Part print with two shaded views. Sizes in mm from the minimum x, y, z corner. A direction names the side the tool comes from. Round coordinates to 2 decimals unless told otherwise and drop trailing zeros. Loops run counter-clockwise (first coordinate to the right, second up) from the corner with the lowest first, then second, coordinate; pieces in that order, holes last. Notation, with made-up numbers: (61.5, 11.5) - (75.5, 11.5) arc R17 ccw to (75.5, 22.5) - close; hole circle Ø8 at (-37, 77). An arc over 180 degrees is marked (long way). Write each question's results on one line, items separated by ' | '. Start each with the question number.
(1) Flat gauge pins, fed straight in: P1, Ø3, axis at x = 16, z = 3.5, coming from the +Y side (1 decimal); P2, Ø1, axis at x = 13.5, y = 4.5, coming from the -Z side; P3, Ø3, axis at y = 3, z = 8, coming from the +X side. Where does each tip first touch, or does it go through?
(2) Drill centre lines: L1, parallel to X at y = 2.25, z = 2; L2, parallel to Y at x = 11, z = 6; L3, parallel to Y at x = 18, z = 7.25. Where is each one in solid material? Low to high.
(3) Cut at A-A, the plane z = 6. List the corners of the cut face in (x, y).
(4) Cut at C-C, the plane y = 1.5. List the corners of the cut face in (x, z).
(5) Cut at D-D, the plane z = 1. List the corners of the cut face in (x, y), then the cut area to 3 significant figures.
(6) Tool access for the marked faces 1 and 2: list every direction of +Z, -Z, +X, -X, +Y, -Y with a clear straight run to the whole face (end or side of a thin tool).
(7) Cut at B-B, the plane x = 36. List the corners of the cut face in (y, z).
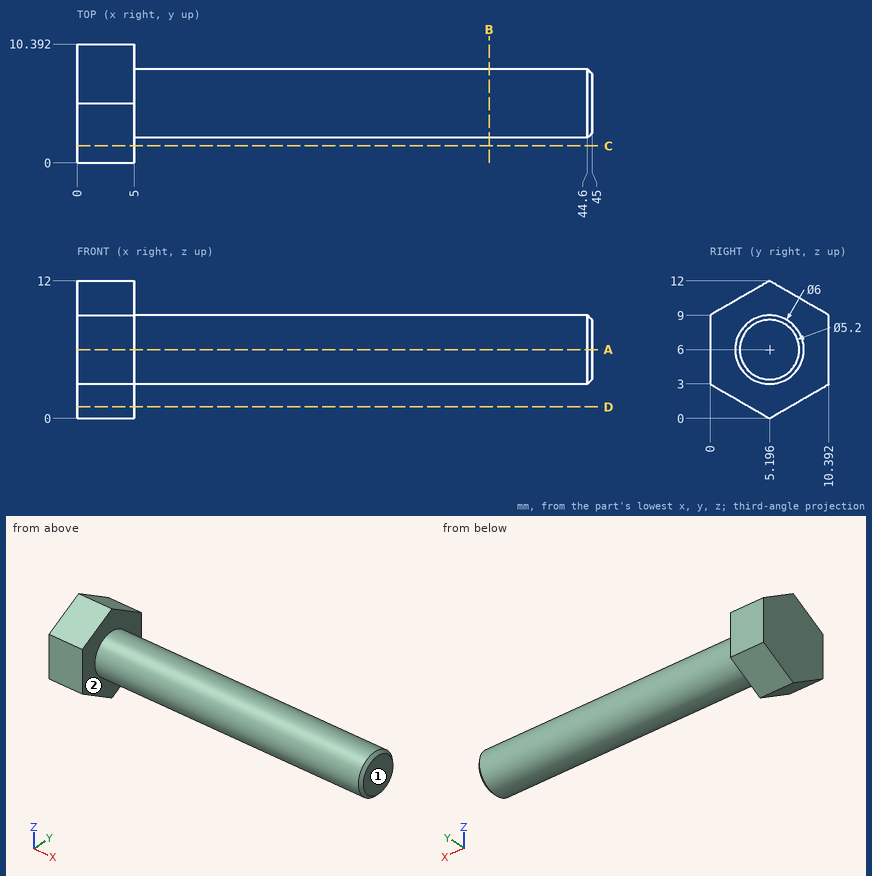
A:
1) P1: y = 8 | P2: z = 3.01 | P3: x = 45
2) L1: 0 to 5 | L2: 2.2 to 8.2 | L3: 2.47 to 7.92
3) outline: (0, 0) - (5, 0) - (5, 2.2) - (44.6, 2.2) - (45, 2.6) - (45, 7.8) - (44.6, 8.2) - (5, 8.2) - (5, 10.39) - (0, 10.39) - close
4) outline: (0, 2.13) - (5, 2.13) - (5, 9.87) - (0, 9.87) - close
5) outline: (0, 3.46) - (5, 3.46) - (5, 6.93) - (0, 6.93) - close | area: 17.3 mm2
6) face 1: +Z, -Z, +X, +Y, -Y | face 2: +X
7) outline: circle Ø6 at (5.2, 6)
